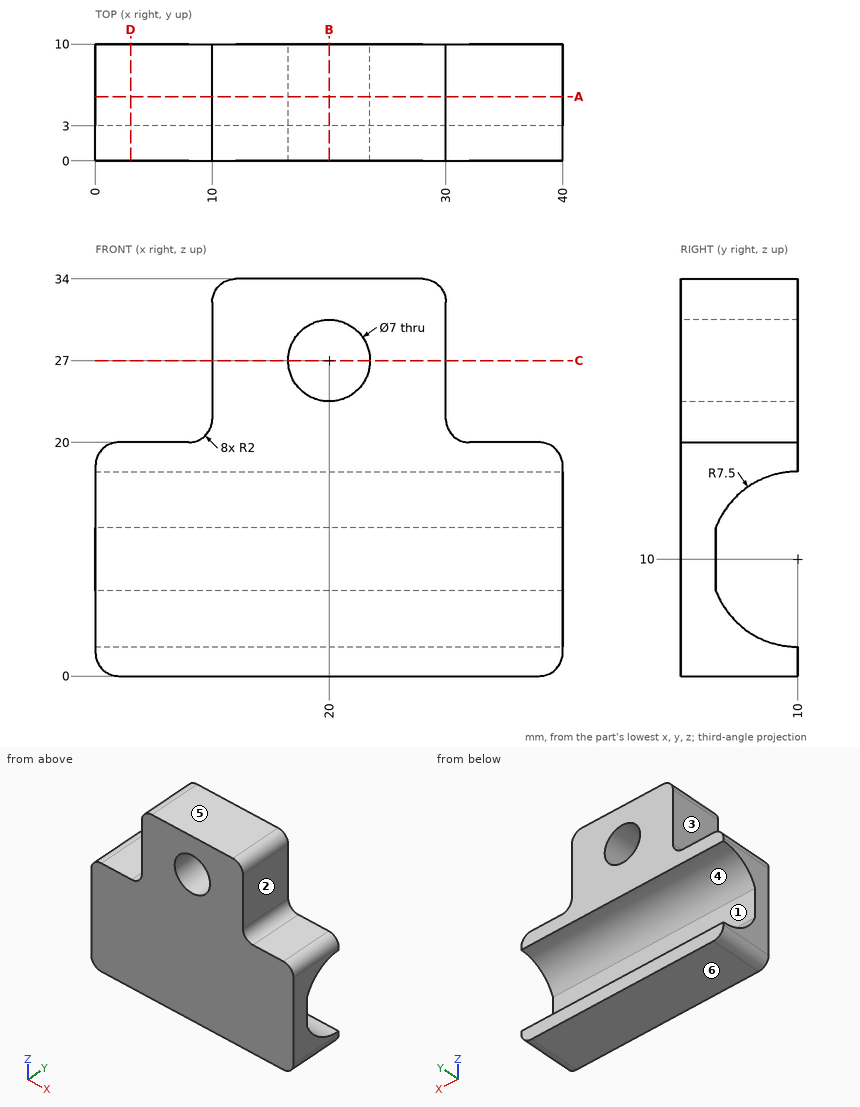
Input: dimensioned drawing with shaded views. Units: mm. Origin: part minimum x, y, z. A direction names the side the tool comes from. Round coordinates to 2 decimals unless told otherwise and drop trailing zeros. Order: outer loops, then holes, each group sorted by start corner. A loop starts at its lowest first (then second) coordinate and runs counter-clockwise, first axis right, second up. Notation, with made-up numbers: (-20, 23) - (1, 23) arc R13 cw to (1, 48) - close; hole circle Ø5 at (-22.75, 12). An arc over 180 degrees is marked (long way). Write item = value, one per line. Start each with the question number.
Q1. Cut plane D-D on x = 3. Return the cut outline in (y, z), and give its area (3 significant figures).
Q2. Access query for the marked faces 1, 2 and 3. Directions: +Z, -Z, +X, -X, +Y, -Y. A direction counts if a zero-diameter tool reaches every point of the face in a straight line with its end or side. Return the directions, or none.
Q3. Cut plane B-B on x = 20. Return the cut outline in (y, z), and give its area (3 significant figures).
Q4. Cut plane C-C on z = 27. Return the cut outline in (x, y), and give its area (3 significant figures).
Q5. Pin query (flat end, axial travel): pin 1 (3 mm diameter, centred on y = 2.5, z = 26.5, fed in from -X); pin 2 (3 mm diameter, centred on x = 5.5, y = 4, fed in from +Z); pin 3 (1.5 mm diameter, centred on y = 8, z = 3.5, fed in from +X); pin 4 (5 mm diameter, centred on x = 33.5, y = 6.5, fed in from +Z). Return the tip coordinate at first contact, or that it passes through.
Q6. Cut plane A-A on y = 5.5. Return the cut outline in (x, z).
Q7. Ray query, line 1 (X direction, y = 6.5, z = 27); line 2 (Z direction, x = 20.5, y = 4.25); line 3 (Z direction, x = 18.5, y = 7.75). Return the intervals inside material, ascending. Write a range as from..to.
Q8. Pull-direction query (Z, two-part tool) for the marked faces 4, 5 and 6; classes: +Z half, -Z half, draft (parallel to the pull), parting line (faces both ways), or undercut.
Outcome:
q1.outline = (0, 0) - (10, 0) - (10, 2.5) arc R7.5 cw to (3, 7.31) - (3, 12.69) arc R7.5 cw to (10, 17.5) - (10, 20) - (0, 20) - close
q1.area = 113 mm^2
q2.face_1 = +X, -X, +Y
q2.face_2 = +Z, +X, +Y, -Y
q2.face_3 = +Z, -X, +Y, -Y
q3.outline = (0, 0) - (10, 0) - (10, 2.5) arc R7.5 cw to (3, 7.31) - (3, 12.69) arc R7.5 cw to (10, 17.5) - (10, 23.5) - (0, 23.5) - close; (0, 30.5) - (10, 30.5) - (10, 34) - (0, 34) - close
q3.area = 183 mm^2
q4.outline = (10, 0) - (16.5, 0) - (16.5, 10) - (10, 10) - close; (23.5, 0) - (30, 0) - (30, 10) - (23.5, 10) - close
q4.area = 130 mm^2
q5.pin_1 = 10
q5.pin_2 = 20
q5.pin_3 = 40
q5.pin_4 = 20.27
q6.outline = (0, 2) arc R2 ccw to (2, 0) - (38, 0) arc R2 ccw to (40, 2) - (40, 4) - (0, 4) - close; (0, 16) - (40, 16) - (40, 18) arc R2 ccw to (38, 20) - (32, 20) arc R2 cw to (30, 22) - (30, 32) arc R2 ccw to (28, 34) - (12, 34) arc R2 ccw to (10, 32) - (10, 22) arc R2 cw to (8, 20) - (2, 20) arc R2 ccw to (0, 18) - close; hole circle Ø7 at (20, 27)
q7.line_1 = 10..16.5, 23.5..30
q7.line_2 = 0..5.18, 14.82..23.54, 30.46..34
q7.line_3 = 0..2.85, 17.15..23.84, 30.16..34
q8.face_4 = undercut
q8.face_5 = +Z half
q8.face_6 = -Z half
